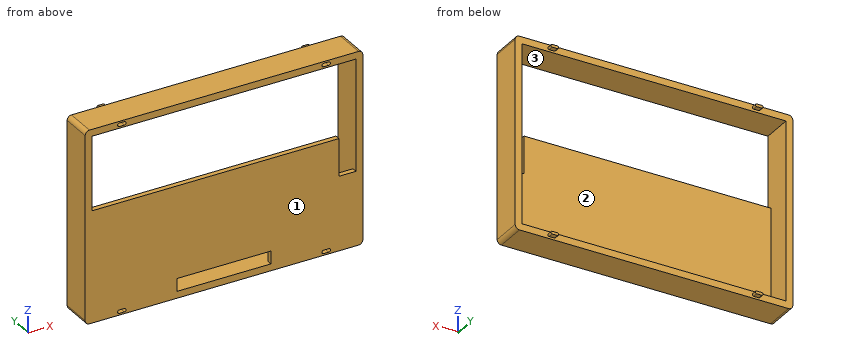
from build123d import *

# Parameters (mm, degrees)
SKETCH3_W            = 163
SKETCH3_H            = 113
BOSS_EXTRUDE2_DEPTH  = 18
SKETCH4_W            = 155
SKETCH4_H            = 105
CUT_EXTRUDE2_DEPTH   = 15
FILLET1_R            = 2.5
SKETCH5_W            = 55
SKETCH5_H            = 7.5
TOPWIRES_DEPTH       = 3
SKETCH6_W            = 155
SKETCH6_H            = 43.5
MOTORWIRES_DEPTH     = 3
CONNECTORHOLES_DEPTH = 3
SKETCH14_W           = 10
SKETCH14_H           = 22
SIDEWIRES_DEPTH      = 3
BOSS_EXTRUDE7_DEPTH  = 3


with BuildPart() as part:
    # Sketch3 → Boss-Extrude2 (new body)
    with BuildSketch(Plane(origin=(0, 0, 0), x_dir=(1, 0, 0), z_dir=(0, 1, 0))):
        Rectangle(SKETCH3_W, SKETCH3_H)
    extrude(amount=BOSS_EXTRUDE2_DEPTH)

    # Sketch4 → Cut-Extrude2 (cut)
    with BuildSketch(Plane(origin=(0, 18, 0), x_dir=(1, 0, 0), z_dir=(0, 1, 0))):
        Rectangle(SKETCH4_W, SKETCH4_H)
    extrude(amount=-CUT_EXTRUDE2_DEPTH, mode=Mode.SUBTRACT)

    # Fillet1
    fillet1_edges = [part.edges().sort_by_distance(p)[0] for p in [
        (81.5, 9, 56.5),
        (-81.5, 9, 56.5),
        (-81.5, 9, -56.5),
        (81.5, 9, -56.5),
    ]]
    fillet(fillet1_edges, radius=FILLET1_R)

    # Sketch5 → TopWires (cut)
    with BuildSketch(Plane(origin=(0, 3, 0), x_dir=(1, 0, 0), z_dir=(0, 1, 0))):
        with Locations((0, 48.75)):
            Rectangle(SKETCH5_W, SKETCH5_H)
    extrude(amount=-TOPWIRES_DEPTH, mode=Mode.SUBTRACT)

    # Sketch6 → MotorWires (cut)
    with BuildSketch(Plane(origin=(0, 3, 0), x_dir=(1, 0, 0), z_dir=(0, 1, 0))):
        with Locations((0, -30.75)):
            Rectangle(SKETCH6_W, SKETCH6_H)
    extrude(amount=-MOTORWIRES_DEPTH, mode=Mode.SUBTRACT)

    # Sketch13 → ConnectorHoles (cut)
    with BuildSketch(Plane(origin=(0, 0, 0), x_dir=(-1, 0, 0), z_dir=(0, -1, 0))):
        with BuildLine():
            Line((61.5, 53.5), (58.5, 53.5))
            ThreePointArc((58.5, 53.5), (57.5, 54.5), (58.5, 55.5))
            Line((58.5, 55.5), (61.5, 55.5))
            ThreePointArc((61.5, 55.5), (62.5, 54.5), (61.5, 53.5))
        make_face()
        with BuildLine():
            Line((-58.5, 53.5), (-61.5, 53.5))
            ThreePointArc((-61.5, 53.5), (-62.5, 54.5), (-61.5, 55.5))
            Line((-61.5, 55.5), (-58.5, 55.5))
            ThreePointArc((-58.5, 55.5), (-57.5, 54.5), (-58.5, 53.5))
        make_face()
        with BuildLine():
            Line((61.5, -55.5), (58.5, -55.5))
            ThreePointArc((58.5, -55.5), (57.5, -54.5), (58.5, -53.5))
            Line((58.5, -53.5), (61.5, -53.5))
            ThreePointArc((61.5, -53.5), (62.5, -54.5), (61.5, -55.5))
        make_face()
        with BuildLine():
            Line((-61.5, -53.5), (-58.5, -53.5))
            ThreePointArc((-58.5, -53.5), (-57.5, -54.5), (-58.5, -55.5))
            Line((-58.5, -55.5), (-61.5, -55.5))
            ThreePointArc((-61.5, -55.5), (-62.5, -54.5), (-61.5, -53.5))
        make_face()
    extrude(amount=-CONNECTORHOLES_DEPTH, mode=Mode.SUBTRACT)

    # Sketch14 → SideWires (cut)
    with BuildSketch(Plane(origin=(0, 3, 0), x_dir=(1, 0, 0), z_dir=(0, 1, 0))):
        with Locations((72.5, 2)):
            Rectangle(SKETCH14_W, SKETCH14_H)
    extrude(amount=-SIDEWIRES_DEPTH, mode=Mode.SUBTRACT)

    # Sketch16 → Boss-Extrude7 (add)
    with BuildSketch(Plane(origin=(0, 18, 0), x_dir=(1, 0, 0), z_dir=(0, 1, 0))):
        with BuildLine():
            Line((61.5, -55.3), (58.5, -55.3))
            ThreePointArc((58.5, -55.3), (57.7, -54.5), (58.5, -53.7))
            Line((58.5, -53.7), (61.5, -53.7))
            ThreePointArc((61.5, -53.7), (62.3, -54.5), (61.5, -55.3))
        make_face()
        with BuildLine():
            Line((-58.5, -55.491947616), (-61.5, -55.491947616))
            ThreePointArc((-61.5, -55.491947616), (-62.3, -54.691947616), (-61.5, -53.891947616))
            Line((-61.5, -53.891947616), (-58.5, -53.891947616))
            ThreePointArc((-58.5, -53.891947616), (-57.7, -54.691947616), (-58.5, -55.491947616))
        make_face()
        with BuildLine():
            Line((-61.5, 55.3), (-58.5, 55.3))
            ThreePointArc((-58.5, 55.3), (-57.7, 54.5), (-58.5, 53.7))
            Line((-58.5, 53.7), (-61.5, 53.7))
            ThreePointArc((-61.5, 53.7), (-62.3, 54.5), (-61.5, 55.3))
        make_face()
        with BuildLine():
            Line((61.5, 53.7), (58.5, 53.7))
            ThreePointArc((58.5, 53.7), (57.7, 54.5), (58.5, 55.3))
            Line((58.5, 55.3), (61.5, 55.3))
            ThreePointArc((61.5, 55.3), (62.3, 54.5), (61.5, 53.7))
        make_face()
    extrude(amount=BOSS_EXTRUDE7_DEPTH)


solid = part.part
The listing builds one solid part. Answer for the finished solid, in the listing's coordinates (mm). Face numbers are marked on the shaded views. A direction names the side the tool comes from. Give positions to 0.01 mm unless a question says otherwise; leave off trailing zeros. Order: outer loops, then holes, each group sorted by start corner. A loop starts at its lowest first (then second) coordinate and runs counter-clockwise, first axis right, second up. Notation, with made-up numbers: (74, -39) -> (123, -39) arc R18 cw to (123, -6) -> close; hole circle Ø5 at (-24.75, 19). An arc over 180 degrees is marked (long way). Put each result on its own line as item: value.
Item 1: A cutting plane is placed at C-C on y = 16. Give the vertices of the cut face in (x, z).
Established:
outline: (-81.5, -54) arc R2.5 ccw to (-79, -56.5) -> (79, -56.5) arc R2.5 ccw to (81.5, -54) -> (81.5, 54) arc R2.5 ccw to (79, 56.5) -> (-79, 56.5) arc R2.5 ccw to (-81.5, 54) -> close; hole (-77.5, -52.5) -> (77.5, -52.5) -> (77.5, 52.5) -> (-77.5, 52.5) -> close
Item 2: A cutting plane is placed at B-B on x = 5.5. Give the vertices of the cut face in (y, z), plus the area to 3 significant figures.
Established:
outline: (0, -56.5) -> (18, -56.5) -> (18, -52.5) -> (0, -52.5) -> close; (0, -45) -> (3, -45) -> (3, 9) -> (0, 9) -> close; (0, 52.5) -> (18, 52.5) -> (18, 56.5) -> (0, 56.5) -> close
area: 306 mm^2
Item 3: Given P1, Ø3.5, axis at x = 60.5, y = 20, coming from the +Z side; P2, Ø0.9, axis at x = -59.5, y = 20, coming from the +Z side; P3, Ø3.5, axis at x = 60, y = 20, coming from the -Z side, each flat-ended and moving along its own axis, determine where each tip first touches the part or whether it passes through.
Established:
P1: stops at z = 55.3
P2: stops at z = 55.49
P3: stops at z = -55.3
Item 4: A cutting plane is placed at A-A on z = -4.5. Give the vertices of the cut face in (x, y), plus the area to 3 significant figures.
Established:
outline: (-81.5, 0) -> (67.5, 0) -> (67.5, 3) -> (-77.5, 3) -> (-77.5, 18) -> (-81.5, 18) -> close; (77.5, 0) -> (81.5, 0) -> (81.5, 18) -> (77.5, 18) -> close
area: 579 mm^2
Item 5: Straight lines are drawn through the part: line 1 (Z direction, x = -74, y = 7); line 2 (X direction, y = 4.5, z = -19); line 3 (Z direction, x = -65.5, y = 2). For each, find the intervals that lie inside material, in ascending order.
Established:
line 1: z = -56.5 to -52.5, 52.5 to 56.5
line 2: x = -81.5 to -77.5, 77.5 to 81.5
line 3: z = -56.5 to 9, 52.5 to 56.5
Item 6: For the marked faces 1, 2 and 3, determine the directions among +Z, -Z, +X, -X, +Y, -Y from which every point of the face is accessible in a straight line to the end or side of a thin tool.
Established:
face 1: +Z, -Z, +X, -X, -Y
face 2: +Y
face 3: +Y, -Y
Item 7: A cutting plane is placed at D-D on x = 70.5. Give the vertices of the cut face in (y, z), plus the area to 4 significant figures.
Established:
outline: (0, -56.5) -> (18, -56.5) -> (18, -52.5) -> (3, -52.5) -> (3, -13) -> (0, -13) -> close; (0, 52.5) -> (18, 52.5) -> (18, 56.5) -> (0, 56.5) -> close
area: 262.5 mm^2
